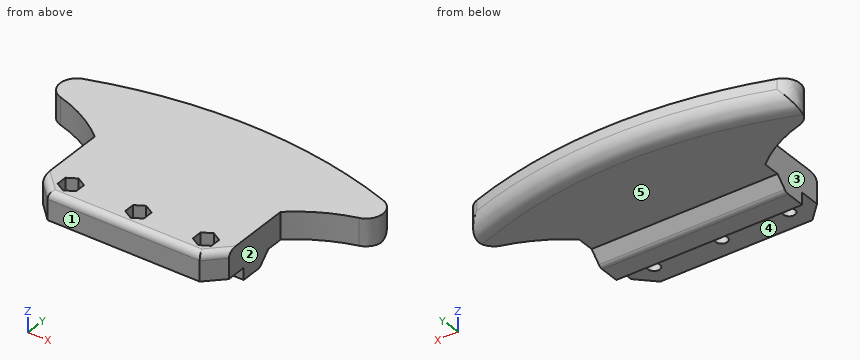
from build123d import *

# Parameters (mm, degrees)
F1_W        = 55
F1_H        = 5
F1_H_2      = 11
F2_DEPTH    = 8
F1_R        = 1.75
F3_DEPTH    = 4
F4_DEPTH    = 3.5
F5_T4_DEPTH = 55
F5_T6_DEPTH = 33.7168298797
F6_R        = 5
F7_R        = 2


# Not quite as in the source:
# - a fillet or chamfer that OpenCascade refuses, or shapes differently, is made with other operations: its cross-section is extruded or revolved along the edge and cut away or added
# - a feature names something its author has since deleted; it is built from what else it names


with BuildPart() as f2:
    # F1 (on Top) → F2 (new body)
    with BuildSketch(Plane.XY):
        with BuildLine():
            Line((-27.5, 10), (-27.5, 0))
            Line((-27.5, 0), (27.5, 0))
            Line((27.5, 0), (27.5, 10))
            ThreePointArc((27.5, 10), (45.1645357284, 19.1976835871), (65.078124404, 19.4843749404))
            ThreePointArc((65.078124404, 19.4843749404), (0, 35.8083822448), (-65.078124404, 19.4843749404))
            ThreePointArc((-65.078124404, 19.4843749404), (-45.1645357284, 19.1976835871), (-27.5, 10))
        make_face()
        with Locations((0, -2.5)):
            Rectangle(F1_W, F1_H)
        with Locations((0, -10.5)):
            Rectangle(F1_W, F1_H_2)
        Polygon((-20, -13.1754264805), (-22.75, -11.5877132403), (-22.75, -8.4122867597), (-20, -6.8245735195), (-17.25, -8.4122867597), (-17.25, -11.5877132403), align=None, mode=Mode.SUBTRACT)
        Polygon((0, -13.1754264805), (-2.75, -11.5877132403), (-2.75, -8.4122867597), (0, -6.8245735195), (2.75, -8.4122867597), (2.75, -11.5877132403), align=None, mode=Mode.SUBTRACT)
        Polygon((20, -13.1754264805), (17.25, -11.5877132403), (17.25, -8.4122867597), (20, -6.8245735195), (22.75, -8.4122867597), (22.75, -11.5877132403), align=None, mode=Mode.SUBTRACT)
    extrude(amount=F2_DEPTH)

    # F1 (on Top) → F3 (join)
    with BuildSketch(Plane.XY):
        Polygon((-22.75, -8.4122867597), (-22.75, -11.5877132403), (-20, -13.1754264805), (-17.25, -11.5877132403), (-17.25, -8.4122867597), (-20, -6.8245735195), align=None)
        with Locations((-20, -10)):
            Circle(F1_R, mode=Mode.SUBTRACT)
        Polygon((-2.75, -8.4122867597), (-2.75, -11.5877132403), (0, -13.1754264805), (2.75, -11.5877132403), (2.75, -8.4122867597), (0, -6.8245735195), align=None)
        with Locations((0, -10)):
            Circle(F1_R, mode=Mode.SUBTRACT)
        Polygon((17.25, -8.4122867597), (17.25, -11.5877132403), (20, -13.1754264805), (22.75, -11.5877132403), (22.75, -8.4122867597), (20, -6.8245735195), align=None)
        with Locations((20, -10)):
            Circle(F1_R, mode=Mode.SUBTRACT)
    extrude(amount=F3_DEPTH)

    # F1 (on Top) → F4 (join)
    with BuildSketch(Plane.XY):
        with Locations((0, -2.5)):
            Rectangle(F1_W, F1_H)
    extrude(amount=-F4_DEPTH)

    # F5: chamfer of 5 on 3 edges, made by hand


with BuildPart() as f5_tool2:
    # F5_s3 → F5_t4 (new body)
    with BuildSketch(Plane.YZ.offset(27.5)):
        Polygon((5, 0), (0, -5), (0, 0), align=None)
    extrude(amount=-F5_T4_DEPTH)

    split(bisect_by=Plane.XY.offset(-3.5), keep=Keep.TOP)


with BuildPart() as f2_1:
    add(f2.part)

    # F5_t1: union F5_tool2
    add(f5_tool2.part)

    # F5_s7 → F5_t6 (cut)
    with BuildSketch(Plane.XY.offset(-12.8584149398)):
        Polygon((-22.5, -16), (-27.5, -11), (-27.5, -16), align=None)
        Polygon((27.5, -11), (22.5, -16), (27.5, -16), align=None)
    extrude(amount=F5_T6_DEPTH, mode=Mode.SUBTRACT)

    # F6
    f6_edges = [f2_1.edges().sort_by_distance(p)[0] for p in [
        (0, 35.808382, 0),
        (-65.078124, 19.484375, 4),
        (65.078124, 19.484375, 4),
    ]]
    fillet(f6_edges, radius=F6_R)

    # F7
    f7_edges = [f2_1.edges().sort_by_distance(p)[0] for p in [
        (0, -16, 8),
        (-25, -13.5, 8),
        (25, -13.5, 8),
        (0, 1.5, -3.5),
    ]]
    fillet(f7_edges, radius=F7_R)


solid = f2_1.part
Verification items for the finished model (mm, model axes). Face numbers are marked on the shaded views. A direction names the side the tool comes from. Coordinates: 2 decimals unless noted, no trailing zeros. Order: outer loops, then holes, each group sorted by start corner. A loop starts at its lowest first (then second) coordinate and runs counter-clockwise, first axis right, second up. Notation, with made-up numbers: M 54.5,82.25 L 81.5,82.25 A21 cw 81.5,113.25 Z; hole C 56.25,81 d1. An arc over 180 degrees is marked long. One line per item, written item: value. Start each with the question number.
Item 1: Thickness scan on probe 1 along Z at (x, y) = (-39, 23); probe 2 along X at (y, z) = (5.5, 7); probe 3 along Y at (x, z) = (-20, 2.65). Record the ranges inside material, lowest first.
Item 2: Access from +Z, -Z, +X, -X, +Y, -Y to the whole of each face (thin tool, end or side, straight path). Record for the marked faces 1, 2, 3, 4 and 5.
Item 3: Sectioned sample at C-C on y = 12. Record the cut outline in (x, z), then the cut area to 3 significant figures.
Item 4: Sectioned sample at B-B on y = -10. Give the number of separate pieces and of enclosed holes in the cut face, then the cut area to 3 significant figures.
Item 5: Sectioned sample at A-A on z = -1.75. Record the cut outline in (x, y), then the cut area to 3 significant figures.
Item 6: Depth check by flat-ended pin: P1, Ø3, axis at y = -9.5, z = 3, coming from the +X side; P2, Ø4, axis at x = -4, y = -9, coming from the -Z side; P3, Ø2.5, axis at y = -9.5, z = 6, coming from the -X side. Enter the tip coordinate at first touch or a pass-through.
Calculated:
1. probe 1: 0 to 8
1. probe 2: -27.5 to 27.5
1. probe 3: -16 to -11.75, -8.25 to 33.76
2. face 1: +Z, -Z, +X, -X, -Y
2. face 2: +Z, -Z, +X, -Y
2. face 3: +Z, -Z, -X, -Y
2. face 4: -Z, +X, -X, -Y
2. face 5: -Z, +X, -X, +Y
3. outline: M -29.99,0 L 29.99,0 L 29.99,8 L -29.99,8 Z
3. area: 480 mm^2
4. separate pieces: 4
4. enclosed holes: 0
4. area: 331 mm^2
5. outline: M -27.5,-5 L 27.5,-5 L 27.5,3.25 L -27.5,3.25 Z
5. area: 454 mm^2
6. P1: x = 27.5
6. P2: z = 0
6. P3: x = -27.5
